Geometry check sheet. Reference: the model listing, model coordinates, mm. Face numbers are marked on the shaded views. A direction names the side the tool comes from. Give positions to 0.01 mm unless a question says otherwise; leave off trailing zeros. Write each loop counter-clockwise with the first axis right and the second up, starting at its lowest first coordinate (ties: lowest second). Pieces come first, ordered by that corner, then holes. Notation, with made-up numbers: (37, -31) -> (56, -31) arc R20 ccw to (56, -9) -> close; hole circle Ø11 at (52.5, -12). An arc over 180 degrees is marked (long way). One line per item, written item: value.
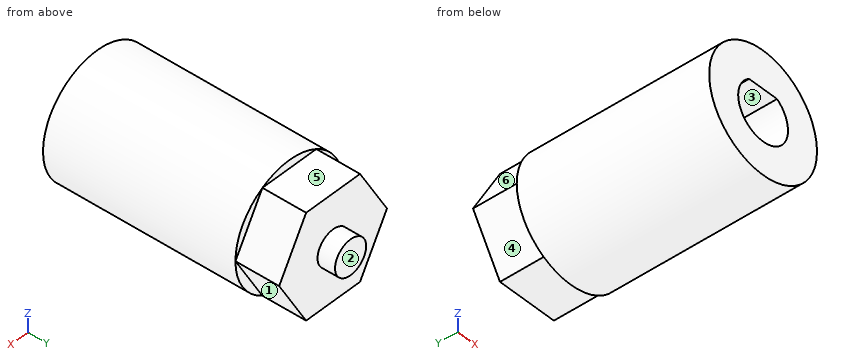
from build123d import *

# Parameters (mm, degrees)
SKETCH1_R           = 2
BOSS_EXTRUDE1_DEPTH = 5
SKETCH1_3_R         = 2
BOSS_EXTRUDE2_DEPTH = 7
SKETCH2_R           = 6.92820323
BOSS_EXTRUDE3_DEPTH = 22


with BuildPart() as part:
    # Sketch1 → Boss-Extrude1 (new body)
    with BuildSketch(Plane(origin=(0, 0, 0), x_dir=(1, 0, 0), z_dir=(0, 1, 0))):
        Circle(SKETCH1_R)
        Polygon((-3.464101615, 6), (-6.92820323, 0), (-3.464101615, -6), (3.464101615, -6), (6.92820323, 0), (3.464101615, 6), align=None)
        Circle(SKETCH1_R, mode=Mode.SUBTRACT)
    extrude(amount=BOSS_EXTRUDE1_DEPTH)

    # Sketch1_3 → Boss-Extrude2 (add)
    with BuildSketch(Plane(origin=(0, 0, 0), x_dir=(1, 0, 0), z_dir=(0, 1, 0))):
        Circle(SKETCH1_3_R)
    extrude(amount=BOSS_EXTRUDE2_DEPTH)

    # Sketch2 → Boss-Extrude3 (add)
    with BuildSketch(Plane.XZ):
        Circle(SKETCH2_R)
        with BuildLine():
            Line((-1.793739111, 2.65), (1.793739111, 2.65))
            ThreePointArc((1.793739111, 2.65), (0, -3.2), (-1.793739111, 2.65))
        make_face(mode=Mode.SUBTRACT)
    extrude(amount=BOSS_EXTRUDE3_DEPTH)


solid = part.part
1) Sectioned sample at D-D on z = -3.75. Record the cut outline in (x, y).
Verdict:
outline: (-5.83, -22) -> (5.83, -22) -> (5.83, 0) -> (4.76, 0) -> (4.76, 5) -> (-4.76, 5) -> (-4.76, 0) -> (-5.83, 0) -> close
2) Depth check by flat-ended pin: pin 1 Ø5.5 at (x, y) = (-1.5, 2.5) entering from +Z; pin 2 Ø1 at (x, z) = (4.5, 2) entering from +Y; pin 3 Ø1 at (y, z) = (-1, -1) entering from -X. Enter the tip coordinate at first touch or a pass-through.
Verdict:
pin 1: z = 6.92
pin 2: y = 5
pin 3: x = -6.91
3) Scan lines: probe 1 along Z at (x, y) = (0, -9); probe 2 along X at (y, z) = (-11.5, 0); probe 3 along Y at (x, z) = (4, -1.25). Record each from-to range of solid material in increasing order.
Verdict:
probe 1: -6.93 to -3.2, 2.65 to 6.93
probe 2: -6.93 to -3.2, 3.2 to 6.93
probe 3: -22 to 5
4) Sectioned sample at A-A on x = 0. Record the cut outline in (y, z), plus the area to 3 significant figures.
Verdict:
outline: (-22, -6.93) -> (0, -6.93) -> (0, -6) -> (5, -6) -> (5, -2) -> (7, -2) -> (7, 2) -> (5, 2) -> (5, 6) -> (0, 6) -> (0, 6.93) -> (-22, 6.93) -> (-22, 2.65) -> (0, 2.65) -> (0, -3.2) -> (-22, -3.2) -> close
area: 244 mm^2
5) Sectioned sample at C-C on y = 3.25. Record the cut outline in (x, z), plus the area to 3 significant figures.
Verdict:
outline: (-6.93, 0) -> (-3.46, -6) -> (3.46, -6) -> (6.93, 0) -> (3.46, 6) -> (-3.46, 6) -> close
area: 125 mm^2
6) Mould release check, pull along Z, two halves, no side actions. Record for the marked faces 1, 2 and 3: released by +Z, released by -Z, zero draft, split by the parting line, or undercut.
Verdict:
face 1: released by -Z
face 2: zero draft
face 3: undercut
7) Sectioned sample at B-B on y = -19.25. Record the cut outline in (x, z).
Verdict:
outline: circle Ø13.86 at (0, 0); hole (-1.79, 2.65) arc R3.2 ccw (long way) to (1.79, 2.65) -> close
8) Tool access check on the marked faces 4, 5 and 6. Record the directions out of +Z, -Z, +X, -X, +Y, -Y that give a thin tool (end or side, any length) a straight path to the whole face; none if there is none.
Verdict:
face 4: -Z, -X, +Y
face 5: +Z, +X, -X, +Y
face 6: +Z, -X, +Y
